For this review, take the finished solid that the model builds, in its own axes (mm). Face numbers are marked on the shaded views. A direction names the side the tool comes from. Coordinates: 2 decimals unless noted, no trailing zeros. Order: outer loops, then holes, each group sorted by start corner. A loop starts at its lowest first (then second) coordinate and runs counter-clockwise, first axis right, second up. Notation, with made-up numbers: M 3,26.5 L 56,26.5 A37 ccw 56,65.5 Z; hole C -31,-18.75 d2. An arc over 180 degrees is marked long. Use CSV: the item, a comma, the result in double quotes.
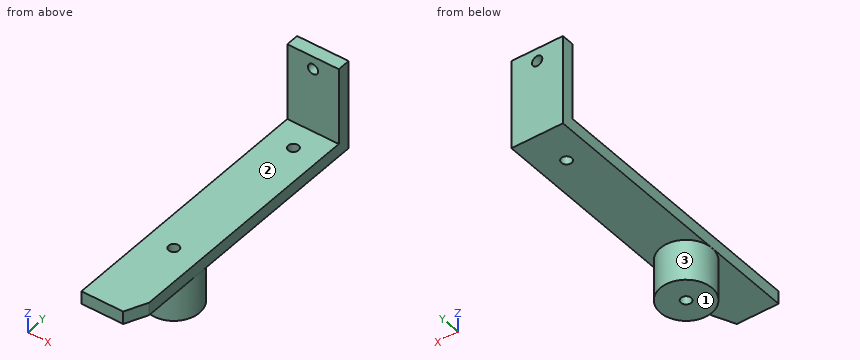
```python
from build123d import *

# Parameters (mm, degrees)
SKETCH1_W           = 12.7
SKETCH1_H           = 3.175
BOSS_EXTRUDE1_DEPTH = 69.85
SKETCH2_W           = 12.7
SKETCH2_H           = 3.175
BOSS_EXTRUDE2_DEPTH = 19.05
SKETCH3_R           = 1.27
CUT_EXTRUDE1_DEPTH  = 71.084124673
SKETCH4_R           = 1.27
CUT_EXTRUDE2_DEPTH  = 73.679071953
SKETCH5_R           = 6.35
SKETCH5_R_2         = 1.27
BOSS_EXTRUDE3_DEPTH = 10.16
CUT_EXTRUDE3_DEPTH  = 73.679071953


with BuildPart() as part:
    # Sketch1 → Boss-Extrude1 (new body)
    with BuildSketch(Plane(origin=(0, 0, 0), x_dir=(1, 0, 0), z_dir=(0, 1, 0))):
        Rectangle(SKETCH1_W, SKETCH1_H)
    extrude(amount=BOSS_EXTRUDE1_DEPTH)

    # Sketch2 → Boss-Extrude2 (add)
    with BuildSketch(Plane.XY.offset(1.5875)):
        with Locations((0, 68.2625)):
            Rectangle(SKETCH2_W, SKETCH2_H)
    extrude(amount=BOSS_EXTRUDE2_DEPTH)

    # Sketch3 → Cut-Extrude1 (cut, through all)
    with BuildSketch(Plane.XZ.offset(-66.675)):
        with Locations(Location((0, 17.4625, 0), (0, 0, 270))):
            Circle(SKETCH3_R)
    extrude(amount=-CUT_EXTRUDE1_DEPTH, mode=Mode.SUBTRACT)

    # Sketch4 → Cut-Extrude2 (cut, through all)
    with BuildSketch(Plane.XY.offset(1.5875)):
        with Locations((0, 21.59)):
            Circle(SKETCH4_R)
        with Locations((0, 60.325)):
            Circle(SKETCH4_R)
    extrude(amount=-CUT_EXTRUDE2_DEPTH, mode=Mode.SUBTRACT)

    # Sketch5 → Boss-Extrude3 (add)
    with BuildSketch(Plane(origin=(0, 0, -1.5875), x_dir=(-1, 0, 0), z_dir=(0, 0, -1))):
        with Locations((0, 21.59)):
            Circle(SKETCH5_R)
        with Locations(Location((0, 21.59, 0), (0, 0, 180))):
            Circle(SKETCH5_R_2, mode=Mode.SUBTRACT)
    extrude(amount=BOSS_EXTRUDE3_DEPTH)

    # Sketch6 → Cut-Extrude3 (cut, through all)
    with BuildSketch(Plane.XY.offset(1.5875)):
        Polygon((3.951482723, 0), (6.35, 5.27166953), (6.35, 0), align=None)
    extrude(amount=-CUT_EXTRUDE3_DEPTH, mode=Mode.SUBTRACT)


solid = part.part
```
Item 1: Add section A-A on x = 0. State how many separate pieces and enclosed holes the cut face has, and give its area (3 significant figures).
Solutions:
separate pieces,"4"
enclosed holes,"0"
area,"361 mm^2"
Item 2: For the marked faces 1, 2 and 3, list the 3-axis set-ups (+Z, -Z, +X, -X, +Y, -Y) from which the entire face can be reached by the end or side of a thin tool; tool diameter is ignored.
Solutions:
face 1,"-Z, +X, -X, +Y, -Y"
face 2,"+Z, +X, -X, -Y"
face 3,"-Z"
Item 3: Add section B-B on z = -4.5. State the section outline as (x, y) points, and give its area (3 significant figures).
Solutions:
outline,"C 0,21.59 d12.7; hole C 0,21.59 d2.54"
area,"122 mm^2"
Item 4: Clearance check with flat-ended pins moving along their axes: pin 1 Ø1 at (x, y) = (3.5, 60.5) entering from +Z; pin 2 Ø6.5 at (x, y) = (2.5, 6) entering from -Z; pin 3 Ø4 at (x, z) = (2, 15) entering from -Y (3 decimals). State where each tip first meets the part, or that it passes through.
Solutions:
pin 1,"z = 1.59"
pin 2,"z = -1.59"
pin 3,"y = 66.675"
Item 5: To check wall thickness, follow line 1 along Y through (x, z) = (0, -0.9) (3 decimals); line 2 along Y through (x, z) = (0, -6); line 3 along Z through (x, y) = (-5.25, 19.5). State the ranges of each line that lie inside material, in increasing order. Write a range as [from, to].
Solutions:
line 1,"[0, 20.32], [22.86, 59.055], [61.595, 69.85]"
line 2,"[15.24, 20.32], [22.86, 27.94]"
line 3,"[-11.75, 1.59]"
Item 6: Add section C-C on y = 43.5. State the section outline as (x, z) points.
Solutions:
outline,"M -6.35,-1.59 L 6.35,-1.59 L 6.35,1.59 L -6.35,1.59 Z"
